CAD build for the part. Positions are in the model's coordinates, mm. Give positions to 0.01 mm unless a question says otherwise; leave off trailing zeros. Loops run counter-clockwise (first coordinate to the right, second up) from the corner with the lowest first, then second, coordinate; pieces in that order, holes last. Notation, with made-up numbers: (38.5, 59.25) -> (70.5, 59.25) arc R16 cw to (70.5, 87.25) -> close; hole circle Ø3 at (-24.5, 25). An arc over 180 degrees is marked (long way). Use one line per item in the form item = value.
```python
from build123d import *

# Parameters (mm, degrees)
F0_R     = 30.95625
F1_DEPTH = 952.5
F6_DEPTH = 9.9724281426


with BuildPart() as f1:
    # F0 (on Right) → F1 (new body)
    with BuildSketch(Plane.YZ):
        Circle(F0_R)
    extrude(amount=F1_DEPTH)

    # F5 (on plane+point) → F6 (cut, up to face)
    with BuildSketch(Plane.XY.offset(21.9838219596)):
        with BuildLine():
            Line((0, 7.9375), (0, 0))
            Line((0, 0), (0, -7.9375))
            Line((0, -7.9375), (119.0625, -7.9375))
            ThreePointArc((119.0625, -7.9375), (111.125, 0), (119.0625, 7.9375))
            Line((119.0625, 7.9375), (0, 7.9375))
        make_face()
        with BuildLine():
            ThreePointArc((119.0625, 7.9375), (111.125, 0), (119.0625, -7.9375))
            ThreePointArc((119.0625, -7.9375), (124.6751600757, -5.6126600757), (127, 0))
            ThreePointArc((127, 0), (124.6751600757, 5.6126600757), (119.0625, 7.9375))
        make_face()
        with BuildLine():
            ThreePointArc((636.5875, -7.9375), (642.2001600757, -5.6126600757), (644.525, 0))
            ThreePointArc((644.525, 0), (642.2001600757, 5.6126600757), (636.5875, 7.9375))
            ThreePointArc((636.5875, 7.9375), (628.65, 0), (636.5875, -7.9375))
        make_face()
        with BuildLine():
            ThreePointArc((636.5875, 7.9375), (642.2001600757, 5.6126600757), (644.525, 0))
            ThreePointArc((644.525, 0), (642.2001600757, -5.6126600757), (636.5875, -7.9375))
            Line((636.5875, -7.9375), (785.8125, -7.9375))
            ThreePointArc((785.8125, -7.9375), (777.875, 0), (785.8125, 7.9375))
            Line((785.8125, 7.9375), (636.5875, 7.9375))
        make_face()
        with BuildLine():
            ThreePointArc((793.75, 0), (791.4251600757, 5.6126600757), (785.8125, 7.9375))
            ThreePointArc((785.8125, 7.9375), (777.875, 0), (785.8125, -7.9375))
            ThreePointArc((785.8125, -7.9375), (791.4251600757, -5.6126600757), (793.75, 0))
        make_face()
    extrude(amount=F6_DEPTH, mode=Mode.SUBTRACT)


solid = f1.part
```
1. Mould opens along X. For faces 1 (the flat face through (0, 0, 0)), 2 (the flat face through (63, 0, 21.984)), 3 (the flat face through (710, 0, 21.984)) say: pulls with the +X half, pulls with the -X half, needs draft (parallel to the pull), parting line crosses it, or undercut.
Result sheet:
face_1 = pulls with the -X half
face_2 = needs draft
face_3 = undercut
2. Cut at B-B, the plane z = -20. Write the cut outline in (x, y).
Result sheet:
outline = (0, -23.63) -> (952.5, -23.63) -> (952.5, 23.63) -> (0, 23.63) -> close
3. Drill centre lines: line 1 (Z direction, x = 331, y = -1); line 2 (Y direction, x = 492.5, z = 2.5); line 3 (Z direction, x = 643.5, y = 1). Where is each one in solid material? Low to high.
Result sheet:
line_1 = -30.94 to 30.94
line_2 = -30.86 to 30.86
line_3 = -30.94 to 21.98
4. Drop flat-ended pins along their axis: P1, Ø8, axis at x = 50, y = 3, coming from the +Z side; P2, Ø6.5, axis at x = 682, z = 27, coming from the +Y side; P3, Ø2.5, axis at x = 46.5, z = 25.5, coming from the +Y side; P4, Ø2, axis at y = 16, z = 0, coming from the -X side. Give the stop position or say it passes through.
Result sheet:
P1 = 21.98
P2 = 19.86
P3 = 19.24
P4 = 0
5. Cut at A-A, the plane x = 696. Write the cut outline in (y, z).
Result sheet:
outline = (-7.94, 21.98) -> (-7.94, 29.92) arc R30.96 ccw (long way) to (7.94, 29.92) -> (7.94, 21.98) -> close
